Source: CAD feature listing. Evaluate the final solid. Frame: model axes, mm. A direction names the side the tool comes from. Give positions to 0.01 mm unless a question says otherwise; leave off trailing zeros. Write each loop counter-clockwise with the first axis right and the second up, starting at its lowest first coordinate (ties: lowest second). Pieces come first, ordered by that corner, then holes.
```python
from build123d import *

# Parameters (mm, degrees)
F0_W     = 1
F0_H     = 54.4
F1_DEPTH = 50
F2_W     = 219.6
F2_H     = 54.4
F3_DEPTH = 1.2
F4_W     = 20
F4_H     = 20
F4_R     = 2.5
F5_DEPTH = 5.2
F6_R     = 3
F7_SIZE  = 3.99999


# Not quite as in the source:
# - a fillet or chamfer is up to 0.001 mm smaller than in the source, because OpenCascade refuses the exact size


with BuildPart() as f1:
    # F0 (on Top) → F1 (new body)
    with BuildSketch(Plane.XY):
        with BuildLine():
            Line((-52.5935795337, -9.6814689702), (-53.5935795337, -9.6814689702))
            ThreePointArc((-53.5935795337, -9.6814689702), (-57.1291134396, -8.2170028761), (-58.5935795337, -4.6814689702))
            Line((-58.5935795337, -4.6814689702), (-58.5935795337, 37.3185310298))
            ThreePointArc((-58.5935795337, 37.3185310298), (-57.1291134396, 40.8540649358), (-53.5935795337, 42.3185310298))
            Line((-53.5935795337, 42.3185310298), (-11.5935795337, 42.3185310298))
            ThreePointArc((-11.5935795337, 42.3185310298), (-8.0580456278, 40.8540649358), (-6.5935795337, 37.3185310298))
            Line((-6.5935795337, 37.3185310298), (-6.5935795337, -4.6814689702))
            ThreePointArc((-6.5935795337, -4.6814689702), (-8.0580456278, -8.2170028761), (-11.5935795337, -9.6814689702))
            Line((-11.5935795337, -9.6814689702), (-12.5935795337, -9.6814689702))
            Line((-12.5935795337, -9.6814689702), (-12.5935795337, -10.8814689702))
            Line((-12.5935795337, -10.8814689702), (-5.3935795337, -10.8814689702))
            Line((-5.3935795337, -10.8814689702), (-5.3935795337, 43.5185310298))
            Line((-5.3935795337, 43.5185310298), (-59.7935795337, 43.5185310298))
            Line((-59.7935795337, 43.5185310298), (-59.7935795337, -10.8814689702))
            Line((-59.7935795337, -10.8814689702), (-52.5935795337, -10.8814689702))
            Line((-52.5935795337, -10.8814689702), (-52.5935795337, -9.6814689702))
        make_face()
        with Locations((-60.2935795337, 16.3185310298)):
            Rectangle(F0_W, F0_H)
        with BuildLine():
            Line((49.0064204663, 43.5185310298), (-5.3935795337, 43.5185310298))
            Line((-5.3935795337, 43.5185310298), (-5.3935795337, -10.8814689702))
            Line((-5.3935795337, -10.8814689702), (1.8064204663, -10.8814689702))
            Line((1.8064204663, -10.8814689702), (1.8064204663, -9.6814689702))
            Line((1.8064204663, -9.6814689702), (0.8064204663, -9.6814689702))
            ThreePointArc((0.8064204663, -9.6814689702), (-2.7291134396, -8.2170028761), (-4.1935795337, -4.6814689702))
            Line((-4.1935795337, -4.6814689702), (-4.1935795337, 37.3185310298))
            ThreePointArc((-4.1935795337, 37.3185310298), (-2.7291134396, 40.8540649358), (0.8064204663, 42.3185310298))
            Line((0.8064204663, 42.3185310298), (42.8064204663, 42.3185310298))
            ThreePointArc((42.8064204663, 42.3185310298), (46.3419543722, 40.8540649358), (47.8064204663, 37.3185310298))
            Line((47.8064204663, 37.3185310298), (47.8064204663, -4.6814689702))
            ThreePointArc((47.8064204663, -4.6814689702), (46.3419543722, -8.2170028761), (42.8064204663, -9.6814689702))
            Line((42.8064204663, -9.6814689702), (41.8064204663, -9.6814689702))
            Line((41.8064204663, -9.6814689702), (41.8064204663, -10.8814689702))
            Line((41.8064204663, -10.8814689702), (49.0064204663, -10.8814689702))
            Line((49.0064204663, -10.8814689702), (49.0064204663, 43.5185310298))
        make_face()
        with BuildLine():
            Line((103.4064204663, 43.5185310298), (49.0064204663, 43.5185310298))
            Line((49.0064204663, 43.5185310298), (49.0064204663, -10.8814689702))
            Line((49.0064204663, -10.8814689702), (56.2064204663, -10.8814689702))
            Line((56.2064204663, -10.8814689702), (56.2064204663, -9.6814689702))
            Line((56.2064204663, -9.6814689702), (55.2064204663, -9.6814689702))
            ThreePointArc((55.2064204663, -9.6814689702), (51.6708865604, -8.2170028761), (50.2064204663, -4.6814689702))
            Line((50.2064204663, -4.6814689702), (50.2064204663, 37.3185310298))
            ThreePointArc((50.2064204663, 37.3185310298), (51.6708865604, 40.8540649358), (55.2064204663, 42.3185310298))
            Line((55.2064204663, 42.3185310298), (97.2064204663, 42.3185310298))
            ThreePointArc((97.2064204663, 42.3185310298), (100.7419543722, 40.8540649358), (102.2064204663, 37.3185310298))
            Line((102.2064204663, 37.3185310298), (102.2064204663, -4.6814689702))
            ThreePointArc((102.2064204663, -4.6814689702), (100.7419543722, -8.2170028761), (97.2064204663, -9.6814689702))
            Line((97.2064204663, -9.6814689702), (96.2064204663, -9.6814689702))
            Line((96.2064204663, -9.6814689702), (96.2064204663, -10.8814689702))
            Line((96.2064204663, -10.8814689702), (103.4064204663, -10.8814689702))
            Line((103.4064204663, -10.8814689702), (103.4064204663, 43.5185310298))
        make_face()
        with BuildLine():
            Line((157.8064204663, 43.5185310298), (103.4064204663, 43.5185310298))
            Line((103.4064204663, 43.5185310298), (103.4064204663, -10.8814689702))
            Line((103.4064204663, -10.8814689702), (110.6064204663, -10.8814689702))
            Line((110.6064204663, -10.8814689702), (110.6064204663, -9.6814689702))
            Line((110.6064204663, -9.6814689702), (109.6064204663, -9.6814689702))
            ThreePointArc((109.6064204663, -9.6814689702), (106.0708865604, -8.2170028761), (104.6064204663, -4.6814689702))
            Line((104.6064204663, -4.6814689702), (104.6064204663, 37.3185310298))
            ThreePointArc((104.6064204663, 37.3185310298), (106.0708865604, 40.8540649358), (109.6064204663, 42.3185310298))
            Line((109.6064204663, 42.3185310298), (151.6064204663, 42.3185310298))
            ThreePointArc((151.6064204663, 42.3185310298), (155.1419543722, 40.8540649358), (156.6064204663, 37.3185310298))
            Line((156.6064204663, 37.3185310298), (156.6064204663, -4.6814689702))
            ThreePointArc((156.6064204663, -4.6814689702), (155.1419543722, -8.2170028761), (151.6064204663, -9.6814689702))
            Line((151.6064204663, -9.6814689702), (150.6064204663, -9.6814689702))
            Line((150.6064204663, -9.6814689702), (150.6064204663, -10.8814689702))
            Line((150.6064204663, -10.8814689702), (157.8064204663, -10.8814689702))
            Line((157.8064204663, -10.8814689702), (157.8064204663, 43.5185310298))
        make_face()
        with Locations((158.3064204663, 16.3185310298)):
            Rectangle(F0_W, F0_H)
    extrude(amount=F1_DEPTH)

    # F2 (on face) → F3 (join)
    with BuildSketch(Plane(origin=(0, 0, 0), x_dir=(1, 0, 0), z_dir=(0, 0, -1))):
        with Locations((49.0064204663, -16.3185310298)):
            Rectangle(F2_W, F2_H)
    extrude(amount=F3_DEPTH)

    # F4 (on face) → F5 (join)
    with BuildSketch(Plane.XZ.offset(-42.3185310298)):
        with Locations((-32.5935795337, 40)):
            Rectangle(F4_W, F4_H)
        with Locations((-38.5935795337, 34)):
            Circle(F4_R, mode=Mode.SUBTRACT)
        with Locations((-32.5935795337, 34)):
            Circle(F4_R, mode=Mode.SUBTRACT)
        with Locations((-26.5935795337, 34)):
            Circle(F4_R, mode=Mode.SUBTRACT)
        with Locations((-38.5935795337, 40)):
            Circle(F4_R, mode=Mode.SUBTRACT)
        with Locations((-32.5935795337, 40)):
            Circle(F4_R, mode=Mode.SUBTRACT)
        with Locations((-26.5935795337, 40)):
            Circle(F4_R, mode=Mode.SUBTRACT)
        with Locations((-38.5935795337, 46)):
            Circle(F4_R, mode=Mode.SUBTRACT)
        with Locations((-32.5935795337, 46)):
            Circle(F4_R, mode=Mode.SUBTRACT)
        with Locations((-26.5935795337, 46)):
            Circle(F4_R, mode=Mode.SUBTRACT)
        with Locations((21.8064204663, 40)):
            Rectangle(F4_W, F4_H)
        with Locations((15.8064204663, 34)):
            Circle(F4_R, mode=Mode.SUBTRACT)
        with Locations((21.8064204663, 34)):
            Circle(F4_R, mode=Mode.SUBTRACT)
        with Locations((27.8064204663, 34)):
            Circle(F4_R, mode=Mode.SUBTRACT)
        with Locations((15.8064204663, 40)):
            Circle(F4_R, mode=Mode.SUBTRACT)
        with Locations((21.8064204663, 40)):
            Circle(F4_R, mode=Mode.SUBTRACT)
        with Locations((27.8064204663, 40)):
            Circle(F4_R, mode=Mode.SUBTRACT)
        with Locations((15.8064204663, 46)):
            Circle(F4_R, mode=Mode.SUBTRACT)
        with Locations((21.8064204663, 46)):
            Circle(F4_R, mode=Mode.SUBTRACT)
        with Locations((27.8064204663, 46)):
            Circle(F4_R, mode=Mode.SUBTRACT)
        with Locations((76.2064204663, 40)):
            Rectangle(F4_W, F4_H)
        with Locations((70.2064204663, 34)):
            Circle(F4_R, mode=Mode.SUBTRACT)
        with Locations((76.2064204663, 34)):
            Circle(F4_R, mode=Mode.SUBTRACT)
        with Locations((82.2064204663, 34)):
            Circle(F4_R, mode=Mode.SUBTRACT)
        with Locations((70.2064204663, 40)):
            Circle(F4_R, mode=Mode.SUBTRACT)
        with Locations((76.2064204663, 40)):
            Circle(F4_R, mode=Mode.SUBTRACT)
        with Locations((82.2064204663, 40)):
            Circle(F4_R, mode=Mode.SUBTRACT)
        with Locations((70.2064204663, 46)):
            Circle(F4_R, mode=Mode.SUBTRACT)
        with Locations((76.2064204663, 46)):
            Circle(F4_R, mode=Mode.SUBTRACT)
        with Locations((82.2064204663, 46)):
            Circle(F4_R, mode=Mode.SUBTRACT)
        with Locations((130.6064204663, 40)):
            Rectangle(F4_W, F4_H)
        with Locations((124.6064204663, 34)):
            Circle(F4_R, mode=Mode.SUBTRACT)
        with Locations((130.6064204663, 34)):
            Circle(F4_R, mode=Mode.SUBTRACT)
        with Locations((136.6064204663, 34)):
            Circle(F4_R, mode=Mode.SUBTRACT)
        with Locations((124.6064204663, 40)):
            Circle(F4_R, mode=Mode.SUBTRACT)
        with Locations((130.6064204663, 40)):
            Circle(F4_R, mode=Mode.SUBTRACT)
        with Locations((136.6064204663, 40)):
            Circle(F4_R, mode=Mode.SUBTRACT)
        with Locations((124.6064204663, 46)):
            Circle(F4_R, mode=Mode.SUBTRACT)
        with Locations((130.6064204663, 46)):
            Circle(F4_R, mode=Mode.SUBTRACT)
        with Locations((136.6064204663, 46)):
            Circle(F4_R, mode=Mode.SUBTRACT)
    extrude(amount=-F5_DEPTH)

    # F6
    f6_edges = [f1.edges().sort_by_distance(p)[0] for p in [
        (-60.79358, -10.881469, 24.4),
        (158.80642, -10.881469, 24.4),
        (-60.79358, 43.518531, 24.4),
        (158.80642, 43.518531, 24.4),
    ]]
    fillet(f6_edges, radius=F6_R)

    # F7 (size 4 in the source; OpenCascade refuses exactly that, so slightly less here)
    f7_edges = [f1.edges().sort_by_distance(p)[0] for p in [
        (130.60642, 43.518531, 30),
        (76.20642, 43.518531, 30),
        (21.80642, 43.518531, 30),
        (-32.59358, 43.518531, 30),
    ]]
    chamfer(f7_edges, length=F7_SIZE)


solid = f1.part
```
1. Pin query (flat end, axial travel): P1, Ø12, axis at x = -32, z = 21.5, coming from the +Y side; P2, Ø4, axis at x = 70.21, z = 34, coming from the -Y side; P3, Ø2.5, axis at x = 130, z = 46.5, coming from the +Y side. Return the tip coordinate at first contact, or that it passes through.
2. Pull-direction query (X, two-part tool) for faces 4 (the flat face through (-35, 47.519, 38)), 5 (the flat face through (-27, 43.519, 46)); classes: pulls with the +X half, pulls with the -X half, needs draft (parallel to the pull), parting line crosses it, or undercut.
3. Access query for faces 1 (the cylindrical face through (22.96, 45.49, 37.78)), 2 (the flat face through (130.47, 45.55, 28.03)), 3 (the cylindrical face through (-57.09, -8.256, 24.65)). Directions: +Z, -Z, +X, -X, +Y, -Y. A direction counts if a zero-diameter tool reaches every point of the face in a straight line with its end or side. Return the directions, or none.
4. Section query A-A (y = 19.5). Return loops of the section in (x, z), plus the area to 3 significant figures.
5. Section query B-B (x = 113). Return loops of the section in (y, z).
6. Line query: probe 1 along X at (y, z) = (34.5, 32.5); probe 2 along X at (y, z) = (41, 8.5); probe 3 along Z at (x, y) = (-37, 6). Output: solid intervals per line, ascending.
The answers:
1. P1: stops at y = 45.02
1. P2: stops at y = 42.32
1. P3: stops at y = 43.52
2. face 4: needs draft
2. face 5: undercut
3. face 1: +Y
3. face 2: -Z, +X, -X, +Y
3. face 3: +Z
4. outline: (-60.79, -1.2) - (158.81, -1.2) - (158.81, 50) - (156.61, 50) - (156.61, 0) - (104.61, 0) - (104.61, 50) - (102.21, 50) - (102.21, 0) - (50.21, 0) - (50.21, 50) - (47.81, 50) - (47.81, 0) - (-4.19, 0) - (-4.19, 50) - (-6.59, 50) - (-6.59, 0) - (-58.59, 0) - (-58.59, 50) - (-60.79, 50) - close
4. area: 844 mm2
5. outline: (-10.88, -1.2) - (43.52, -1.2) - (43.52, 50) - (42.32, 50) - (42.32, 0) - (-10.88, 0) - close
6. probe 1: x = -60.79 to -58.59, -6.59 to -4.19, 47.81 to 50.21, 102.21 to 104.61, 156.61 to 158.81
6. probe 2: x = -60.75 to -56.98, -8.21 to -2.58, 46.19 to 51.82, 100.59 to 106.22, 154.99 to 158.77
6. probe 3: z = -1.2 to 0
